Part model, mm, in its own coordinate system. Give positions to 0.01 mm unless a question says otherwise; leave off trailing zeros. Order: outer loops, then holes, each group sorted by start corner. A loop starts at its lowest first (then second) coordinate and runs counter-clockwise, first axis right, second up. Notation, with made-up numbers: M 82.5,54.25 L 99.5,54.25 A17 ccw 99.5,70.25 Z; hole C 80,-9.5 d11. An arc over 180 degrees is marked long. Return JSON: item names as keys, results as strings.
Autodesk Inventor part; units mm, degrees
ref_plane "YZ Plane" through (0, 0, 0) normal (1, 0, 0) x (0, 1, 0)
ref_plane "XZ Plane" through (0, 0, 0) normal (0, 1, 0) x (-1, 0, 0)
ref_plane "XY Plane" through (0, 0, 0) normal (0, 0, 1) x (1, 0, 0)
sketch "Sketch1" plane through (0, 0, 0) normal (0, 0, 1) x (1, 0, 0)
  line L0 (0, 0) -> (-41.402, 0)
  line L1 (-41.402, 0) -> (-177.8, 93.599)
  line L2 (-177.8, 93.599) -> (-177.8, 135.001)
  line L3 (-177.8, 135.001) -> (0, 135.001)
  line L4 (0, 135.001) -> (0, 0)
  circle A0 centre (-20.701, 12.7) radius 3.3655
  circle A1 centre (-20.701, 63.5) radius 3.3655
  circle A2 centre (-20.701, 114.3) radius 3.3655
  circle A3 centre (-71.501, 114.3) radius 3.3655
  circle A4 centre (-122.301, 114.3) radius 3.3655
  circle A5 centre (-173.101, 114.3) radius 3.3655
  dimension "d0" = 41.402
  dimension "d1" = 41.402
  dimension "d2" = 177.8
  dimension "d3" = 135.001
  dimension "d4" = 6.731
  dimension "d6" = 20.701
  dimension "d9" = 50.8
  dimension "d14" = 20.701
  dimension "d15" = 20.701
  dimension "d16" = 50.8
  dimension "d17" = 12.7
  dimension "d20" = 50.8
  dimension "d25" = 4.699
extrude "Extrusion1" add sketch "Sketch1" along normal blind 2.286
fillet "Fillet1" radius 3.175 5 edges at (0, 135.001, 1.143) (0, 0, 1.143) (-41.402, 0, 1.143) (-177.8, 93.599, 1.143) (-177.8, 135.001, 1.143)
sketch "Sketch2" plane through (0, 0, 2.286) normal (0, 0, 1) x (1, 0, 0)
  point P0 (0, 0)
properties part number "super5" material "Aluminum 6061"
Q1. Band-saw the part on B-B (z = 0.4). Give the number of separate pieces and of enclosed holes in the cut face, then the cut area to 3 significant figures.
Established:
{"separate pieces": "1", "enclosed holes": "6", "area": "17,400 mm²"}
Q2. Two-plate mould, pull along X, no slides. Class faces 1 (the flat face through (-108.38, 45.96, 1.13)), 2 (the flat face through (-70, 83, 2.286)), 3 (the cylindrical face through (-21.431, 117.585, 1.127)): +X half, -X half, draft (parallel to the pull), parting line (faces both ways), or undercut.
Established:
{"face 1": "-X half", "face 2": "draft", "face 3": "undercut"}
Q3. Band-saw the part on D-D (y = 12.7). Give the cut face in (x, z), then the cut area to 3 significant figures.
Established:
{"outline": "M -59.91,0 L -24.07,0 L -24.07,2.29 L -59.91,2.29 Z; M -17.34,0 L 0,0 L 0,2.29 L -17.34,2.29 Z", "area": "122 mm²"}
Q4. Band-saw the part on A-A (y = 114.3). Give the cut face in (x, z), then the cut area to 3 significant figures.
Established:
{"outline": "M -177.8,0 L -176.47,0 L -176.47,2.29 L -177.8,2.29 Z; M -169.74,0 L -125.67,0 L -125.67,2.29 L -169.74,2.29 Z; M -118.94,0 L -74.87,0 L -74.87,2.29 L -118.94,2.29 Z; M -68.14,0 L -24.07,0 L -24.07,2.29 L -68.14,2.29 Z; M -17.34,0 L 0,0 L 0,2.29 L -17.34,2.29 Z", "area": "345 mm²"}
Q5. Probe line 1 along X through (y, z) = (116, 0.45); line 2 along X through (y, z) = (113, 0.35); line 3 along Y through (x, z) = (-64, 1.8). List the from-to ranges inside material, lowest first.
Established:
{"line 1": "x = -177.8 to -176.01, -170.2 to -125.21, -119.4 to -74.41, -68.6 to -23.61, -17.8 to 0", "line 2": "x = -177.8 to -176.21, -170 to -125.41, -119.2 to -74.61, -68.4 to -23.81, -17.6 to 0", "line 3": "y = 15.51 to 135"}
Q6. Band-saw the part on C-C (y = 63.5). Give the cut face in (x, z).
Established:
{"outline": "M -133.94,0 L -24.07,0 L -24.07,2.29 L -133.94,2.29 Z; M -17.34,0 L 0,0 L 0,2.29 L -17.34,2.29 Z"}
Q7. Pin check, flat tip, straight feed: pin 1 (6 mm diameter, centred on x = -20.701, y = 12.7, fed in from +Z). Stop position of the tip, or through.
Established:
{"pin 1": "passes through"}
